The model under review builds one solid part; all positions refer to its coordinate system, in mm. A direction names the side the tool comes from. Round coordinates to 2 decimals unless told otherwise and drop trailing zeros. Write each loop counter-clockwise with the first axis right and the second up, starting at its lowest first coordinate (ties: lowest second). Pieces come first, ordered by that corner, then holes. Notation, with made-up numbers: (65, 4) -> (72, 4) arc R13 cw to (72, 28) -> close; hole circle Ø8 at (-15, 83.25). An arc over 180 degrees is marked (long way). Return JSON: item names as keys, results as strings. Group by question number.
1. Take a section at C-C, the plane x = 8. Write out the cut boundary in (y, z), then the cut area to 3 significant figures.
2. Mouldability with a two-part tool opening along Z and no side actions: class faces 1 (the cylindrical face through (23.715, 0.301, 0.126)), 2 (the cylindrical face through (23.715, 11.154, 8.699)), 3 (the cylindrical face through (-3, 1, 0)), 4 (the cylindrical face through (5.07, 2.699, -3.285)) as pulls with the +Z half, pulls with the -Z half, needs draft (parallel to the pull), parting line crosses it, or undercut.
3. Clearance check with flat-ended pins moving along their axes: P1, Ø7, axis at y = 13, z = 0, coming from the +X side; P2, Ø4, axis at y = 20.5, z = -1.5, coming from the -X side; P3, Ø10, axis at x = -2, y = 12, coming from the -Z side; P4, Ø4, axis at x = 2.5, z = 3, coming from the +Y side. State where each tip first meets the part, or that it passes through.
4. Take a section at B-B, the plane y = 13. Write out the cut boundary in (x, z), then the cut area to 3 significant figures.
5. Take a section at A-A, the plane z = 0. Write out the cut boundary in (x, y).
6. Take a section at D-D, the plane y = 17.5. Write out the cut boundary in (x, z).
7. For line 1 along Y through (x, z) = (21.8, 0); line 2 along Z through (x, y) = (4, 1.5); line 3 along X through (y, z) = (11, 6.5), list the stretches that pass through material, from the lowest coordinate up. Write a range as from..to.
8. Tool access review of faces 5 (the cylindrical face through (4.93, 2.699, 3.285)), 6 (the flat face through (18, 10, 2)), 7 (the cylindrical face through (18.301, 12.633, 8.715)), 8 (the flat face through (5, 1, -3)): name each direction out of +Z, -Z, +X, -X, +Y, -Y from which nothing blocks a thin tool from reaching the whole face with its end or side.
from build123d import *

# Parameters (mm, degrees)
BOSS_EXTRUDE1_DEPTH = 3
CUT_EXTRUDE1_DEPTH  = 3
SKETCH3_W           = 6
SKETCH3_H           = 18
BOSS_EXTRUDE2_DEPTH = 20
FILLET1_R           = 1
FILLET3_R           = 1
FILLET6_R           = 1
SKETCH4_R           = 3
CUT_EXTRUDE2_DEPTH  = 42.218927691
FILLET7_R           = 1


with BuildPart() as part:
    # Sketch1 → Boss-Extrude1 (new body)
    with BuildSketch(Plane(origin=(0, 0, 0), x_dir=(1, 0, 0), z_dir=(0, 1, 0))):
        with BuildLine():
            Line((0, 9), (24, 9))
            Line((24, 9), (24, -9))
            Line((24, -9), (0, -9))
            ThreePointArc((0, -9), (-9, 0), (0, 9))
        make_face()
    extrude(amount=BOSS_EXTRUDE1_DEPTH)

    # Sketch2 → Cut-Extrude1 (cut)
    with BuildSketch(Plane(origin=(0, 3, 0), x_dir=(1, 0, 0), z_dir=(0, 1, 0))):
        with BuildLine():
            Line((0, 3), (10, 3))
            Line((10, 3), (10, -3))
            Line((10, -3), (0, -3))
            ThreePointArc((0, -3), (-3, 0), (0, 3))
        make_face()
    extrude(amount=-CUT_EXTRUDE1_DEPTH, mode=Mode.SUBTRACT)

    # Sketch3 → Boss-Extrude2 (add)
    with BuildSketch(Plane(origin=(0, 3, 0), x_dir=(1, 0, 0), z_dir=(0, 1, 0))):
        with Locations((21, 0)):
            Rectangle(SKETCH3_W, SKETCH3_H)
    extrude(amount=BOSS_EXTRUDE2_DEPTH)

    # Fillet1
    fillet1_edges = [part.edges().sort_by_distance(p)[0] for p in [
        (24, 0, 0),
        (24, 11.5, 9),
        (24, 11.5, -9),
    ]]
    fillet(fillet1_edges, radius=FILLET1_R)

    # Fillet3
    fillet3_edges = [part.edges().sort_by_distance(p)[0] for p in [
        (23.707106781, 23, 8.707106781),
        (23.707106781, 23, -8.707106781),
        (18, 23, 0),
        (20.5, 23, -9),
        (20.5, 23, 9),
        (24, 23, 0),
        (18, 13, 9),
        (18, 13, -9),
    ]]
    fillet(fillet3_edges, radius=FILLET3_R)

    # Fillet6
    fillet6_edges = [part.edges().sort_by_distance(p)[0] for p in [
        (-3, 3, 0),
        (5, 3, 3),
        (5, 3, -3),
    ]]
    fillet(fillet6_edges, radius=FILLET6_R)

    # Sketch4 → Cut-Extrude2 (cut, through all)
    with BuildSketch(Plane(origin=(24, 0, 0), x_dir=(0, 0, -1), z_dir=(1, 0, 0))):
        with Locations((0, 13)):
            Circle(SKETCH4_R)
    extrude(amount=-CUT_EXTRUDE2_DEPTH, mode=Mode.SUBTRACT)

    # Fillet7
    fillet7_edges = [part.edges().sort_by_distance(p)[0] for p in [
        (24, 13, 3),
    ]]
    fillet(fillet7_edges, radius=FILLET7_R)


solid = part.part
Output:
{
 "1": {"outline": "(0, -9) -> (3, -9) -> (3, -4) arc R1 ccw to (2, -3) -> (0, -3) -> close; (0, 3) -> (2, 3) arc R1 ccw to (3, 4) -> (3, 9) -> (0, 9) -> close", "area": "35.6 mm^2"},
 "2": {"face 1": "needs draft", "face 2": "pulls with the +Z half", "face 3": "undercut", "face 4": "undercut"},
 "3": {"P1": "stops at x = 23.87", "P2": "stops at x = 18", "P3": "passes through", "P4": "stops at y = 3"},
 "4": {"outline": "(18, -8) arc R1 ccw to (19, -9) -> (23, -9) arc R1 ccw to (24, -8) -> (24, -4) arc R1 ccw to (23, -3) -> (18, -3) -> close; (18, 3) -> (23, 3) arc R1 ccw to (24, 4) -> (24, 8) arc R1 ccw to (23, 9) -> (19, 9) arc R1 ccw to (18, 8) -> close", "area": "70.7 mm^2"},
 "5": {"outline": "(-9, 0) -> (-3, 0) -> (-3, 2) arc R1 ccw to (-4, 3) -> (-9, 3) -> close; (10, 0) -> (23, 0) arc R1 ccw to (24, 1) -> (24, 9) arc R1 ccw to (23, 10) -> (18, 10) -> (18, 3) -> (10, 3) -> close; (18, 16) -> (23, 16) arc R1 ccw to (24, 17) -> (24, 22) arc R1 ccw to (23, 23) -> (19, 23) arc R1 ccw to (18, 22) -> close"},
 "6": {"outline": "(18, -8) arc R1 ccw to (19, -9) -> (23, -9) arc R1 ccw to (24, -8) -> (24, 8) arc R1 ccw to (23, 9) -> (19, 9) arc R1 ccw to (18, 8) -> close"},
 "7": {"line 1": "y = 0..10, 16..23", "line 2": "z = -9..-3, 3..9", "line 3": "x = 18..24"},
 "8": {"face 5": "+Y", "face 6": "+Z, -Z, -X, +Y", "face 7": "+Z, -X, +Y", "face 8": "+Y, -Y"}
}
